from build123d import *

# Parameters (mm, degrees)
F0_W     = 50
F0_H     = 10
F1_DEPTH = 120
F2_R     = 5
F3_DEPTH = 15
F5_DEPTH = 5
F6_R     = 19.99999


# Not quite as in the source:
# - a fillet or chamfer is up to 0.001 mm smaller than in the source, because OpenCascade refuses the exact size


with BuildPart() as f1:
    # F0 (on Top) → F1 (new body)
    with BuildSketch(Plane.XY):
        Rectangle(F0_W, F0_H)
    extrude(amount=F1_DEPTH)

    # F2 (on face) → F3 (join)
    with BuildSketch(Plane.XZ.offset(5)):
        with Locations((0, 100)):
            Circle(F2_R)
    extrude(amount=F3_DEPTH)

    # F4 (on face) → F5 (join)
    with BuildSketch(Plane(origin=(0, 0, 0), x_dir=(1, 0, 0), z_dir=(0, 0, -1))):
        with BuildLine():
            ThreePointArc((-3.84e-08, -5), (3.5355338924, -3.5355339195), (5, 0))
            ThreePointArc((5, 0), (3.5355339085, 3.5355339034), (7.2e-09, 5))
            ThreePointArc((7.2e-09, 5), (-5, 2.28e-08), (-3.84e-08, -5))
        make_face()
    extrude(amount=F5_DEPTH)

    # F6 (radius 20 in the source; OpenCascade refuses exactly that, so slightly less here)
    f6_edges = [f1.edges().sort_by_distance(p)[0] for p in [
        (25, 0, 0),
        (-25, 0, 0),
        (-25, 0, 120),
        (25, 0, 120),
    ]]
    fillet(f6_edges, radius=F6_R)


solid = f1.part
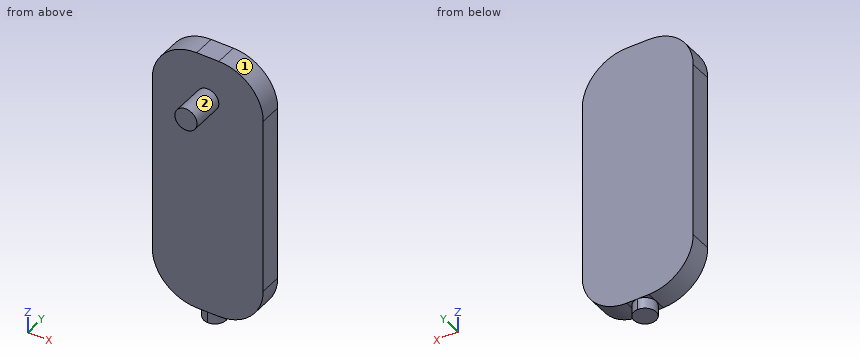
Build history of the part. All positions in model axes, mm. Face numbers are marked on the shaded views. A direction names the side the tool comes from. Round coordinates to 2 decimals unless told otherwise and drop trailing zeros. Loops run counter-clockwise (first coordinate to the right, second up) from the corner with the lowest first, then second, coordinate; pieces in that order, holes last. Notation, with made-up numbers: (5.25, -8.75) -> (16.25, -8.75) arc R13 cw to (16.25, 15.25) -> close; hole circle Ø2 at (24.5, -21). An arc over 180 degrees is marked (long way). Answer in a Markdown table with one row per item.
Item 1: Which spindle directions (+Z, -Z, +X, -X, +Y, -Y) get a long thin tool onto all of the face, cutting with end or side? Do the marked faces 1 and 2. Say none if no direction does.
Answers below:
| item | result |
|---|---|
| face 1 | +Z, +X, +Y, -Y |
| face 2 | -Y |
Item 2: Pin check, flat tips, straight feed: pin 1 (10 mm diameter, centred on x = -6.5, y = -6.5, fed in from -Z); pin 2 (6 mm diameter, centred on x = -7.5, z = 9, fed in from -Y). Stop position of each tip, or through.
Answers below:
| item | result |
|---|---|
| pin 1 | stops at z = -5 |
| pin 2 | stops at y = -5 |
Item 3: Drill centre lines: L1, parallel to Y at x = 21.5, z = 19; L2, parallel to Z at x = 0.5, y = -17; L3, parallel to X at y = -5.5, z = 103. Where is each one in solid material? Low to high. Write a range as [from, to].
Answers below:
| item | result |
|---|---|
| L1 | y = [-5, 5] |
| L2 | z = [95.03, 104.97] |
| L3 | x = [-4, 4] |
Item 4: Saw through at A-A (z = 39). Write the cut outline in (x, y), and give its area (3 significant figures).
Answers below:
| item | result |
|---|---|
| outline | (-25, -5) -> (25, -5) -> (25, 5) -> (-25, 5) -> close |
| area | 500 mm² |
Item 5: Saw through at B-B (x = 16.5). Write the cut outline in (y, z).
Answers below:
| item | result |
|---|---|
| outline | (-5, 3.64) -> (5, 3.64) -> (5, 116.36) -> (-5, 116.36) -> close |
Item 6: Saw through at C-C (y = -13.5). Write the cut outline in (x, z), and give its area (3 significant figures).
Answers below:
| item | result |
|---|---|
| outline | circle Ø10 at (0, 100) |
| area | 78.5 mm² |
